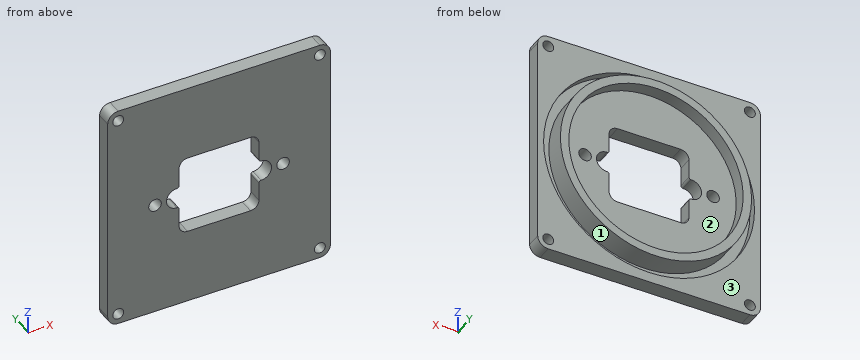
Autodesk Inventor part; units mm, degrees
ref_plane "作業平面1" through (-1.8524, -8.2893, -39.454) normal (0, 1, 0) x (1, 0, 0)
ref_plane "YZ Plane" through (0, 0, 0) normal (1, 0, 0) x (0, 1, 0)
ref_plane "XZ Plane" through (0, 0, 0) normal (0, 1, 0) x (-1, 0, 0)
ref_plane "作業平面1" through (-1.8524, -8.2893, -39.454) normal (0, 1, 0) x (1, 0, 0)
sketch "スケッチ1" plane through (-1.8524, -8.2893, -39.454) normal (0, 1, 0) x (1, 0, 0)
  line L0 (9.655, 16.755) -> (9.655, 15.8775)
  arc A0 (6.855, 15.8775) -> (9.655, 15.8775) centre (8.255, 8.255) ccw
  line L1 (6.855, 15.8775) -> (6.855, 16.755)
  line L2 (6.855, 16.755) -> (0.755, 16.755)
  arc A1 (0.755, 16.755) -> (-0.245, 15.755) centre (0.755, 15.755) ccw
  line L3 (-0.245, 15.755) -> (-0.245, 10.155)
  line L4 (-0.245, 10.155) -> (-1.745, 10.155)
  arc A2 (-1.745, 10.155) -> (-1.745, 6.355) centre (-1.745, 8.255) ccw
  line L5 (-1.745, 6.355) -> (-0.245, 6.355)
  line L6 (-0.245, 6.355) -> (-0.245, 0.755)
  arc A3 (-0.245, 0.755) -> (0.755, -0.245) centre (0.755, 0.755) ccw
  line L7 (0.755, -0.245) -> (15.755, -0.245)
  arc A4 (15.755, -0.245) -> (16.755, 0.755) centre (15.755, 0.755) ccw
  line L8 (16.755, 0.755) -> (16.755, 6.355)
  line L9 (16.755, 6.355) -> (18.255, 6.355)
  arc A5 (18.255, 6.355) -> (18.255, 10.155) centre (18.255, 8.255) ccw
  line L10 (18.255, 10.155) -> (16.755, 10.155)
  line L11 (16.755, 10.155) -> (16.755, 15.755)
  arc A6 (16.755, 15.755) -> (15.755, 16.755) centre (15.755, 15.755) ccw
  line L12 (15.755, 16.755) -> (9.655, 16.755)
  circle A7 centre (-1.745, 8.255) radius 0.9
  circle A8 centre (18.255, 8.255) radius 0.9
  line L13 (-15.745, -19.245) -> (32.255, -19.245)
  line L14 (34.755, -16.745) -> (34.755, 33.255)
  line L15 (32.255, 35.755) -> (-15.745, 35.755)
  line L16 (-18.245, 33.255) -> (-18.245, -16.745)
  line L17 (-18.245, -19.245) -> (34.755, 35.755) construction
  line L18 (34.755, -19.245) -> (-18.245, 35.755) construction
  arc A9 (-15.745, 35.755) -> (-18.245, 33.255) centre (-15.745, 33.255) ccw
  arc A10 (34.755, 33.255) -> (32.255, 35.755) centre (32.255, 33.255) ccw
  arc A11 (32.255, -19.245) -> (34.755, -16.745) centre (32.255, -16.745) ccw
  arc A12 (-18.245, -16.745) -> (-15.745, -19.245) centre (-15.745, -16.745) ccw
  circle A13 centre (-15.745, 33.255) radius 1.3
  circle A14 centre (32.255, 33.255) radius 1.3
  circle A15 centre (32.255, -16.745) radius 1.3
  circle A16 centre (-15.745, -16.745) radius 1.3
  line L19 (32.255, -16.745) -> (-15.745, -16.745) construction
  line L20 (-15.745, -16.745) -> (-15.745, 33.255) construction
  line L21 (-15.745, 33.255) -> (32.255, 33.255) construction
  line L22 (32.255, 33.255) -> (32.255, -16.745) construction
  line L23 (32.255, -16.745) -> (-15.745, 33.255) construction
  line L24 (-15.745, -16.745) -> (32.255, 33.255) construction
  line L25 (6.855, 16.755) -> (9.655, 16.755)
  circle A17 centre (-6.985, 8.255) radius 1.5
  circle A18 centre (18.26, 8.26) radius 1.27
  circle A19 centre (23.495, 8.255) radius 1.5
  arc A20 (-1.745, 10.755) -> (-1.745, 5.755) centre (-1.745, 8.255) ccw
  arc A21 (18.26, 5.76) -> (18.26, 10.76) centre (18.26, 8.26) ccw
  arc A22 (17.755, 15.755) -> (15.755, 17.755) centre (15.755, 15.755) ccw
  arc A23 (15.755, -1.245) -> (17.755, 0.755) centre (15.755, 0.755) ccw
  arc A24 (-1.245, 0.755) -> (0.755, -1.245) centre (0.755, 0.755) ccw
  arc A25 (0.755, 17.755) -> (-1.245, 15.755) centre (0.755, 15.755) ccw
  line L26 (0.755, 17.755) -> (15.755, 17.755)
  line L27 (17.755, 15.755) -> (17.755, 10.76)
  line L28 (17.755, 10.76) -> (18.26, 10.76)
  line L29 (17.755, 0.755) -> (17.755, 5.76)
  line L30 (17.755, 5.76) -> (18.26, 5.76)
  line L31 (15.755, -1.245) -> (0.755, -1.245)
  line L32 (-1.245, 0.755) -> (-1.245, 5.755)
  line L33 (-1.245, 5.755) -> (-1.745, 5.755)
  line L34 (-1.745, 10.755) -> (-1.245, 10.755)
  line L35 (-1.245, 10.755) -> (-1.245, 15.755)
  point P0 (1.8524, -39.454)
  dimension "d2" = 2.5
  dimension "d3" = 2.6
  dimension "d4" = 50
  dimension "d5" = 48
  dimension "d15" = 2.5
  dimension "d16" = 2
extrude "押し出し1" add sketch "スケッチ1" along normal blind 3.5 contours A12 L16 A9 L15 A10 L14 A11 L13
sketch "スケッチ2" plane through (-1.8524, -4.7893, -39.454) normal (0, 1, 0) x (1, 0, 0)
  arc A0 (32.255, -19.245) -> (34.755, -16.745) centre (32.255, -16.745) ccw
  line L0 (34.755, -16.745) -> (34.755, 33.255)
  arc A1 (34.755, 33.255) -> (32.255, 35.755) centre (32.255, 33.255) ccw
  line L1 (32.255, 35.755) -> (-15.745, 35.755)
  arc A2 (-15.745, 35.755) -> (-18.245, 33.255) centre (-15.745, 33.255) ccw
  line L2 (-18.245, 33.255) -> (-18.245, -16.745)
  arc A3 (-18.245, -16.745) -> (-15.745, -19.245) centre (-15.745, -16.745) ccw
  line L3 (-15.745, -19.245) -> (32.255, -19.245)
  circle A4 centre (-15.745, -16.745) radius 1.3
  circle A5 centre (32.255, -16.745) radius 1.3
  circle A6 centre (32.255, 33.255) radius 1.3
  circle A7 centre (-15.745, 33.255) radius 1.3
  circle A8 centre (8.255, 8.255) radius 25.1
  circle A9 centre (8.255, 8.255) radius 22.75
  circle A10 centre (8.255, 8.255) radius 20.75
  point P0 (1.8524, -39.454)
  dimension "d8" = 50.2
  dimension "d9" = 45.5
  dimension "d10" = 2
extrude "押し出し2" add sketch "スケッチ2" along normal blind 3 contours A9
extrude "押し出し3" cut sketch "スケッチ2" against normal blind 2 contours A8
fillet "フィレット1" radius 0.5 4 edges at (-3.0974, -6.5393, -50.209) (-3.0974, -6.5393, -45.209) (15.9026, -6.5393, -50.214) (15.9026, -6.5393, -45.214)
properties part number "Camera_Mount"
For this review, take the finished solid that the model builds, in its own axes (mm). Face numbers are marked on the shaded views. Give positions to 0.01 mm unless a question says otherwise; leave off trailing zeros. Loops run counter-clockwise (first coordinate to the right, second up) from the corner with the lowest first, then second, coordinate; pieces in that order, holes last. Notation, with made-up numbers: M 41.5,72 L 97.5,72 A25 ccw 97.5,86 Z; hole C -34,-14.75 d9. An arc over 180 degrees is marked long. Answer as a JSON object with one key per item and string values. Group by question number.
Q1. Add section A-A on x = -2. Give the boundary of the cut face in (y, z), and give its area (3 significant figures).
Q2. Mouldability with a two-part tool opening along Z and no side actions: class the marked faces 1, 2 and 3 as +Z half, -Z half, draft (parallel to the pull), parting line (faces both ways), or undercut.
Q3. Add section B-B on z = -56. Give the boundary of the cut face in (x, y).
Q4. Add section D-D on y = -4. Give the boundary of the cut face in (x, z).
Q5. Add section C-C on z = -34.5. Give the boundary of the cut face in (x, y).
Q6. Insertion check: P1, Ø1.6, axis at x = 30.4, z = -72.71, coming from the +Y side; P2, Ø3, axis at x = 9, y = -3, coming from the +Z side; P3, Ø1.5, axis at x = -12.5, y = -3, coming from the +Z side; P4, Ø1, axis at x = 7.5, y = -2.5, coming from the -Z side. Each pin has a flat end and moves straight along its axis. Give the tip position at first contact, or say it passes through.
Q7. For probe 1 along Z at (x, y) = (6, -5.75); probe 2 along Z at (x, y) = (13.5, -6); probe 3 along Z at (x, y) = (6.5, -4.5), list the stretches that pass through material, from the lowest coordinate up. Write a range as [from, to].
Checked values:
{
 "1": {"outline": "M -8.29,-75.21 L -4.79,-75.21 L -4.79,-71.36 L -6.79,-71.36 L -6.79,-68.85 L -1.79,-68.85 L -1.79,-66.68 L -4.79,-66.68 L -4.79,-56.99 L -8.29,-56.99 Z; M -8.29,-38.42 L -4.79,-38.42 L -4.79,-28.74 L -1.79,-28.74 L -1.79,-26.57 L -6.79,-26.57 L -6.79,-24.06 L -4.79,-24.06 L -4.79,-20.21 L -8.29,-20.21 Z", "area": "130 mm²"},
 "2": {"face 1": "undercut", "face 2": "undercut", "face 3": "draft"},
 "3": {"outline": "M -20.1,-8.29 L -2.93,-8.29 L -2.93,-4.79 L -12.62,-4.79 L -12.62,-1.79 L -14.78,-1.79 L -14.78,-6.79 L -17.29,-6.79 L -17.29,-4.79 L -20.1,-4.79 Z; M 15.74,-8.29 L 32.9,-8.29 L 32.9,-4.79 L 30.09,-4.79 L 30.09,-6.79 L 27.59,-6.79 L 27.59,-1.79 L 25.42,-1.79 L 25.42,-4.79 L 15.74,-4.79 Z"},
 "4": {"outline": "C 6.4,-47.71 d45.5; hole C 6.4,-47.71 d41.5"},
 "5": {"outline": "M -20.1,-8.29 L 32.9,-8.29 L 32.9,-4.79 L 27.75,-4.79 L 27.75,-6.79 L 24.93,-6.79 L 24.93,-1.79 L 22.41,-1.79 L 22.41,-4.79 L -9.6,-4.79 L -9.6,-1.79 L -12.12,-1.79 L -12.12,-6.79 L -14.94,-6.79 L -14.94,-4.79 L -20.1,-4.79 Z"},
 "6": {"P1": "through", "P2": "z = -24.99", "P3": "z = -34", "P4": "z = -70.45"},
 "7": {"probe 1": "[-75.21, -72.81], [-70.46, -57.21], [-38.21, -24.96], [-22.61, -20.21]", "probe 2": "[-75.21, -71.78], [-69.32, -57.21], [-38.21, -26.09], [-23.63, -20.21]", "probe 3": "[-70.46, -68.46], [-26.96, -24.96]"}
}
